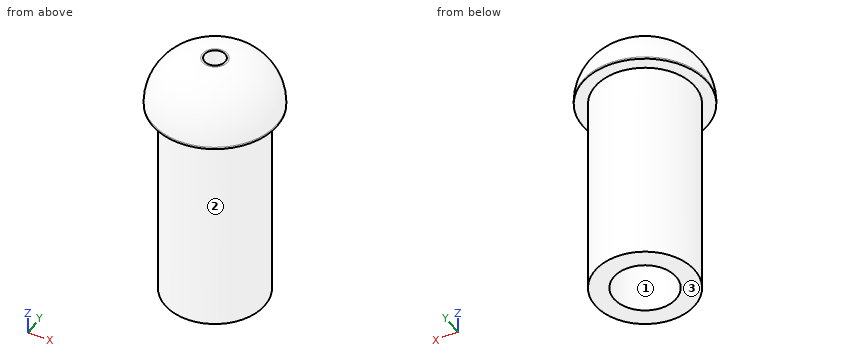
from build123d import *

# Parameters (mm, degrees)
SKETCH_R      = 4.8
SKETCH_R_2    = 3
PAD_DEPTH     = 20
SKETCH001_R   = 6
SKETCH001_R_2 = 1
PAD001_DEPTH  = 5
FILLET_R      = 4.8


with BuildPart() as part:
    # Sketch → Pad (new body)
    with BuildSketch(Plane.XY):
        Circle(SKETCH_R)
        Circle(SKETCH_R_2, mode=Mode.SUBTRACT)
    extrude(amount=PAD_DEPTH)

    # Sketch001 (on Face4 of Pad) → Pad001 (join)
    with BuildSketch(Plane.XY.offset(20)):
        Circle(SKETCH001_R)
        Circle(SKETCH001_R_2, mode=Mode.SUBTRACT)
    extrude(amount=PAD001_DEPTH)

    # Fillet
    fillet_edges = [part.edges().sort_by_distance(p)[0] for p in [
        (-6, 0, 25),
    ]]
    fillet(fillet_edges, radius=FILLET_R)


solid = part.part
Work out the finished part from the listing and answer in its coordinate system (mm). Face numbers are marked on the shaded views. Round coordinates to 2 decimals unless told otherwise and drop trailing zeros. Write each loop counter-clockwise with the first axis right and the second up, starting at its lowest first coordinate (ties: lowest second). Pieces come first, ordered by that corner, then holes. Notation, with made-up numbers: (-33, -3.5) -> (19, -3.5) arc R26 ccw to (19, 31.5) -> close; hole circle Ø10 at (80, 42.5). An arc over 180 degrees is marked (long way). Write each question's results on one line, items separated by ' | '.
Item 1: Flat-ended cylindrical pins translate along their axes: P1, Ø6, axis at y = -1, z = 14.5, coming from the +X side; P2, Ø6, axis at x = 4, z = 20, coming from the +Y side; P3, Ø1.8, axis at x = 0, y = 1, coming from the -Z side. Find the tip coordinate at first contact, or state that the pin passes through.
Result set:
P1: x = 4.8 | P2: y = 5.92 | P3: z = 20
Item 2: The mould has two halves that part along X. Classify the marked faces 1, 2 and 3: +X half, -X half, draft (parallel to the pull), parting line (faces both ways), or undercut.
Result set:
face 1: undercut | face 2: parting line | face 3: draft
Item 3: A cutting plane is placed at A-A, the plane z = 9. Determine the outline of the cut face in (x, y), plus the area to 3 significant figures.
Result set:
outline: circle Ø9.6 at (0, 0); hole circle Ø6 at (0, 0) | area: 44.1 mm^2
Item 4: Find the intervals of material crossed by line 1 along Y through (x, z) = (0, 9.25); line 2 along Y through (x, z) = (-1, 6.25); line 3 along X through (y, z) = (1.75, 9.25), in increasing order. Write a range as [from, to].
Result set:
line 1: [-4.8, -3], [3, 4.8] | line 2: [-4.69, -2.83], [2.83, 4.69] | line 3: [-4.47, -2.44], [2.44, 4.47]
